from build123d import *

# Parameters (mm, degrees)
F0_R     = 50.8
F0_R_2   = 25.4
F1_DEPTH = 6.35
F2_R     = 28.575
F2_R_2   = 25.4
F3_DEPTH = 152.4
F4_W     = 12.7
F4_H     = 51.4328
F5_DEPTH = 158.751


with BuildPart() as f1:
    # F0 (on Top) → F1 (new body)
    with BuildSketch(Plane.XY):
        Circle(F0_R)
        Circle(F0_R_2, mode=Mode.SUBTRACT)
    extrude(amount=F1_DEPTH)

    # F2 (on face) → F3 (join)
    with BuildSketch(Plane.XY.offset(6.35)):
        Circle(F2_R)
        Circle(F2_R_2, mode=Mode.SUBTRACT)
    extrude(amount=F3_DEPTH)

    # F4 (on face) → F5 (cut, through all)
    with BuildSketch(Plane(origin=(0, 0, 0), x_dir=(1, 0, 0), z_dir=(0, 0, -1))):
        with Locations((0, -39.142372)):
            Rectangle(F4_W, F4_H)
    extrude(amount=-F5_DEPTH, mode=Mode.SUBTRACT)


solid = f1.part
Geometry check sheet. Reference: the model listing, model coordinates, mm. A direction names the side the tool comes from. Give positions to 0.01 mm unless a question says otherwise; leave off trailing zeros. Write each loop counter-clockwise with the first axis right and the second up, starting at its lowest first coordinate (ties: lowest second). Pieces come first, ordered by that corner, then holes. Notation, with made-up numbers: M -27,23.25 L 16,23.25 A16 cw 16,38.25 Z; hole C 40.5,28 d11. An arc over 180 degrees is marked long. Answer as CSV lines item,"result". Start each with the question number.
Q1. Section check B-B, the plane x = -22. Record the cut outline in (y, z).
Q2. Section check D-D, the plane x = 0. Record the cut outline in (y, z) (3 decimals), then the cut area to 3 significant figures.
Q3. Tool access check on faces 1 (the face through (-2.145, -50.755, 3.131)), 2 (the face through (6.35, 27, 61)). Record the directions out of +Z, -Z, +X, -X, +Y, -Y that give a thin tool (end or side, any length) a straight path to the whole face; none if there is none.
Q4. Section check A-A, the plane y = 0. Record the cut outline in (x, z) (3 decimals), then the cut area to 3 significant figures.
Q5. Material ranges on L1, parallel to X at y = 0, z = 73.5 (3 decimals); L2, parallel to Y at x = 0, z = 108 (3 decimals); L3, parallel to Z at x = -16, y = 27, recorded low to high.
Q6. Section check C-C, the plane z = 47.5. Record the cut outline in (x, y) (3 decimals), then the cut area to 3 significant figures.
Q7. Release check for a two-part mould opening along X. For faces 3 (the face through (-6.35, 27, 61)), 4 (the face through (22, -22, 6.35)), 5 (the face through (-1.17, -28.55, 81.48)) record: pulls with the +X half, pulls with the -X half, needs draft (parallel to the pull), parting line crosses it, or undercut.
Q8. Go/stop test with flat-tipped pins: pin 1 (4 mm diameter, centred on y = 28, z = 117, fed in from +X); pin 2 (5 mm diameter, centred on x = 38, y = -6, fed in from +Z); pin 3 (5 mm diameter, centred on x = 8.5, z = 46.5, fed in from +Y); pin 4 (2 mm diameter, centred on x = 12.5, y = -28.5, fed in from -Z). Record where each tip stops, or that it passes through.
Geometry says:
1,outline,"M -45.79,0 L -12.69,0 L -12.69,158.75 L -18.24,158.75 L -18.24,6.35 L -45.79,6.35 Z; M 12.69,0 L 45.79,0 L 45.79,6.35 L 18.24,6.35 L 18.24,158.75 L 12.69,158.75 Z"
2,outline,"M -50.8,0 L -25.4,0 L -25.4,158.75 L -28.575,158.75 L -28.575,6.35 L -50.8,6.35 Z"
2,area,"645 mm^2"
3,face 1,"+Z, -Z"
3,face 2,"+Z, -Z, +Y"
4,outline,"M -50.8,0 L -25.4,0 L -25.4,158.75 L -28.575,158.75 L -28.575,6.35 L -50.8,6.35 Z; M 25.4,0 L 50.8,0 L 50.8,6.35 L 28.575,6.35 L 28.575,158.75 L 25.4,158.75 Z"
4,area,"1,290 mm^2"
5,L1,"-28.575 to -25.4, 25.4 to 28.575"
5,L2,"-28.575 to -25.4"
5,L3,"0 to 6.35"
6,outline,"M -6.35,24.593 L -6.35,27.861 A28.575 ccw long 6.35,27.861 L 6.35,24.593 A25.4 cw long Z"
6,area,"498 mm^2"
7,face 3,"undercut"
7,face 4,"needs draft"
7,face 5,"parting line crosses it"
8,pin 1,"x = 11.85"
8,pin 2,"z = 6.35"
8,pin 3,"y = 27.86"
8,pin 4,"z = 0"
